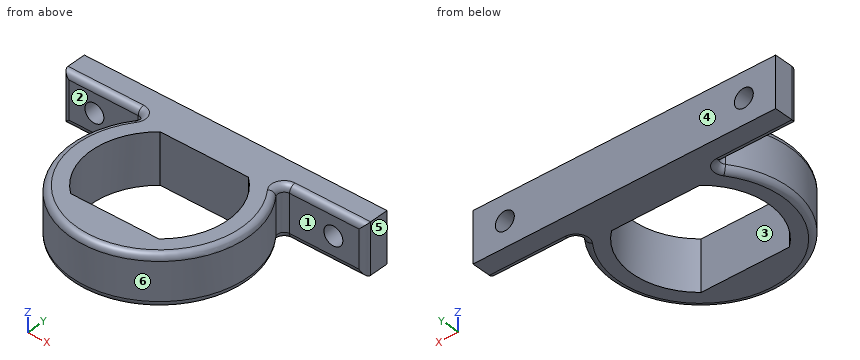
from build123d import *

# Parameters (mm, degrees)
SALIENTE_EXTRUIR1_DEPTH = 8
CORTAR_EXTRUIR1_DEPTH   = 29.91366459
REDONDEO1_R             = 1
CROQUIS3_R              = 1.5
CORTAR_EXTRUIR2_DEPTH   = 35.871191548


with BuildPart() as part:
    # Croquis1 → Saliente-Extruir1 (new body)
    with BuildSketch(Plane.XY):
        with BuildLine():
            Line((0, 14), (-24, 14))
            Line((-24, 14), (-24, 10))
            Line((-24, 10), (-9.797958971, 10))
            ThreePointArc((-9.797958971, 10), (0, -14), (9.797958971, 10))
            Line((9.797958971, 10), (24, 10))
            Line((24, 10), (24, 14))
            Line((24, 14), (0, 14))
        make_face()
    extrude(amount=SALIENTE_EXTRUIR1_DEPTH)

    # Croquis2 → Cortar-Extruir1 (cut, through all)
    with BuildSketch(Plane.XY.offset(8)):
        with BuildLine():
            Line((-7, 8.224354078), (7, 8.224354078))
            ThreePointArc((7, 8.224354078), (10.8, 0), (7, -8.224354078))
            Line((7, -8.224354078), (-7, -8.224354078))
            ThreePointArc((-7, -8.224354078), (-10.8, 0), (-7, 8.224354078))
        make_face()
    extrude(amount=-CORTAR_EXTRUIR1_DEPTH, mode=Mode.SUBTRACT)

    # Redondeo1
    redondeo1_edges = [part.edges().sort_by_distance(p)[0] for p in [
        (16.898979486, 10, 8),
        (-24, 10, 4),
        (-9.797958971, 10, 4),
        (9.797958971, 10, 4),
        (24, 10, 4),
        (0, -14, 8),
        (-16.898979486, 10, 8),
        (-16.898979486, 10, 0),
        (0, -14, 0),
        (16.898979486, 10, 0),
    ]]
    fillet(redondeo1_edges, radius=REDONDEO1_R)

    # Croquis3 → Cortar-Extruir2 (cut, through all)
    with BuildSketch(Plane(origin=(0, 10, 0), x_dir=(-1, 0, 0), z_dir=(0, -1, 0))):
        with Locations(Location((18.949489743, -4, 0), (0, 0, 90))):
            Circle(CROQUIS3_R)
        with Locations(Location((-18.949489743, -4, 0), (0, 0, 90))):
            Circle(CROQUIS3_R)
    extrude(amount=-CORTAR_EXTRUIR2_DEPTH, mode=Mode.SUBTRACT)


solid = part.part
Verification items for the finished model (mm, model axes). Face numbers are marked on the shaded views. A direction names the side the tool comes from. Round coordinates to 2 decimals unless told otherwise and drop trailing zeros. Loops run counter-clockwise (first coordinate to the right, second up) from the corner with the lowest first, then second, coordinate; pieces in that order, holes last. Notation, with made-up numbers: M 62.5,62 L 118.5,62 A36 cw 118.5,98 Z; hole C 72,1.5 d9. An arc over 180 degrees is marked long. Write each question's results on one line, items separated by ' | '.
1) Section check B-B on z = 4. Record the boundary of the cut face in (x, y).
Checks:
outline: M -24,11 A1 ccw -23,10 L -20.45,10 L -20.45,14 L -24,14 Z; M -17.45,10 L -12,10 A1 cw -11.2,8.4 A14 ccw long 11.2,8.4 A1 cw 12,10 L 17.45,10 L 17.45,14 L -17.45,14 Z; M 20.45,10 L 23,10 A1 ccw 24,11 L 24,14 L 20.45,14 Z; hole M -7,-8.22 L 7,-8.22 A10.8 ccw 7,8.22 L -7,8.22 A10.8 ccw Z
2) Scan lines: L1, parallel to X at y = 12.15, z = 4; L2, parallel to Y at x = 22.5, z = 3.75; L3, parallel to Y at x = -5.5, z = 5.5. Record each from-to range of solid material in increasing order. Write a range as from..to.
Checks:
L1: x = -24..-20.45, -17.45..17.45, 20.45..24 | L2: y = 10..14 | L3: y = -12.87..-8.22, 8.22..14
3) Section check D-D on x = -19.5. Record the boundary of the cut face in (y, z), then the cut area to 3 significant figures.
Checks:
outline: M 10,1 A1 ccw 11,0 L 14,0 L 14,2.6 L 10,2.6 Z; M 10,5.4 L 14,5.4 L 14,8 L 11,8 A1 ccw 10,7 Z | area: 20.4 mm2
4) Section check C-C on z = 6. Record the boundary of the cut face in (x, y), then the cut area to 3 significant figures.
Checks:
outline: M -24,11 A1 ccw -23,10 L -12,10 A1 cw -11.2,8.4 A14 ccw long 11.2,8.4 A1 cw 12,10 L 23,10 A1 ccw 24,11 L 24,14 L -24,14 Z; hole M -7,-8.22 L 7,-8.22 A10.8 ccw 7,8.22 L -7,8.22 A10.8 ccw Z | area: 438 mm2
5) Mould release check, pull along Y, two halves, no side actions. Record for the marked faces 4, 5 and 6: released by +Y, released by -Y, zero draft, split by the parting line, or undercut.
Checks:
face 4: released by +Y | face 5: zero draft | face 6: undercut
6) Gauge pin test, flat ends, axial feed: P1, Ø4, axis at y = 4.5, z = 6.5, coming from the -X side (3 decimals); P2, Ø2.5, axis at x = -18.95, z = 4, coming from the -Y side; P3, Ø3, axis at x = -16, z = 5, coming from the -Y side. Record the tip position at first contact, or that the pin passes through.
Checks:
P1: stops at x = -13.775 | P2: passes through | P3: stops at y = 10
7) Section check A-A on x = 0. Record the boundary of the cut face in (y, z).
Checks:
outline: M -14,1 A1 ccw -13,0 L -8.22,0 L -8.22,8 L -13,8 A1 ccw -14,7 Z; M 8.22,0 L 14,0 L 14,8 L 8.22,8 Z
8) Access from +Z, -Z, +X, -X, +Y, -Y to the whole of each face (thin tool, end or side, straight path). Record for the marked faces 1, 2 and 3.
Checks:
face 1: +Z, -Z, +X | face 2: +Z, -Z, -X | face 3: +Z, -Z
